Autodesk Inventor part; units mm, degrees
ref_plane "YZ Plane" through (0, 0, 0) normal (1, 0, 0) x (0, 1, 0)
ref_plane "XZ Plane" through (0, 0, 0) normal (0, 1, 0) x (-1, 0, 0)
ref_plane "XY Plane" through (0, 0, 0) normal (0, 0, 1) x (1, 0, 0)
sketch "Szkic1" plane through (0, 0, 0) normal (0, 0, 1) x (1, 0, 0)
  line L0 (0, 0) -> (2.8284, 0)
  line L1 (2.8284, 0) -> (-27.1716, 30)
  line L2 (-27.1716, 30) -> (-27.1716, 27.1716)
  line L3 (-27.1716, 27.1716) -> (0, 0)
  line L4 (-27.1716, 30) -> (-28, 30)
  line L5 (-28, 30) -> (-28, 28)
  line L6 (-28, 28) -> (-27.1716, 28)
  line L7 (-27.1716, 28) -> (-27.1716, 30)
  line L8 (-28, 28) -> (-27.1716, 27.1716)
  dimension "d1" = 30
  dimension "d3" = 45
  dimension "d20" = 2
  dimension "d21" = 2
extrude "Wyciągnięcie proste1" add sketch "Szkic1" along normal blind 196.178
sketch "Szkic4" plane through (-28, 28, 0) normal (-1, 0, 0) x (0, 0, 1)
  line L0 (0, 0) -> (0, -28)
  line L1 (0, 2) -> (196.178, 2)
  line L2 (0, -28) -> (0, 2)
  line L3 (0, 2) -> (30, 2)
  line L4 (30, 2) -> (0, -28)
  line L5 (98.089, 2) -> (98.089, -28) construction
  line L6 (196.178, 0) -> (196.178, -28)
  line L7 (196.178, -28) -> (196.178, 2)
  line L8 (196.178, 2) -> (166.178, 2)
  line L9 (166.178, 2) -> (196.178, -28)
  dimension "d22" = 45
extrude "Wyciągnięcie proste3" cut sketch "Szkic4" against normal through all
sketch "Szkic5" plane through (2.8284, 0, 0) normal (0.7071, 0.7071, 0) x (-0.7071, 0.7071, 0)
  line L0 (41.598, 28) -> (41.598, 168.178) construction
  line L1 (41.598, 98.089) -> (0, 98.089) construction
  line L2 (0, 0) -> (0, 196.178) construction
  point P0 (2, 0)
  point P1 (36.298, 155.089)
  point P2 (36.298, 41.089)
  point P3 (25.298, 167.089)
  point P4 (25.298, 29.089)
  dimension "d25" = 57
  dimension "d26" = 5.3
  dimension "d34" = 69
  dimension "d35" = 16.3
hole "Otwór2" at (-22.8381, 25.6665, 155.089) at (-22.8381, 25.6665, 41.089) at (-15.0599, 17.8884, 167.089) at (-15.0599, 17.8884, 29.089) direction (-0.7071, -0.7071, 0) diameter 3.2 end through all countersink diameter 6.9 countersink angle 84.225
properties part number "Tyl2"
Model file for the job. Use its own axes, mm. Round coordinates to 2 decimals unless told otherwise and drop trailing zeros. Write each loop counter-clockwise with the first axis right and the second up, starting at its lowest first coordinate (ties: lowest second). Pieces come first, ordered by that corner, then holes. Notation, with made-up numbers: (47.25, 8.25) -> (67.25, 8.25) arc R26 cw to (67.25, 44.25) -> close; hole circle Ø3 at (55.5, -30.5). An arc over 180 degrees is marked (long way). Answer as CSV lines item,"result".
1. Slice it at C-C, the plane x = -8.5. List the corners of the cut face in (y, z).
Resolved:
outline,"(8.5, 8.5) -> (11.33, 11.33) -> (11.33, 184.85) -> (8.5, 187.68) -> close"
2. Slice it at A-A, the plane z = 96. List the corners of the cut face in (x, y).
Resolved:
outline,"(-28, 28) -> (0, 0) -> (2.83, 0) -> (-27.17, 30) -> (-28, 30) -> close"
3. Drill centre lines: line 1 (X direction, y = 7.5, z = 112.5); line 2 (X direction, y = 27, z = 63.5); line 3 (Y direction, x = -8.5, z = 31). Where is each one in solid material? Low to high.
Resolved:
line 1,"-7.5 to -4.67"
line 2,"-27 to -24.17"
line 3,"8.5 to 11.33"
4. Slice it at B-B, the plane y = 12.5. List the corners of the cut face in (x, z), plus the area to 3 significant figures.
Resolved:
outline,"(-12.5, 12.5) -> (-9.67, 12.5) -> (-9.67, 183.68) -> (-12.5, 183.68) -> close"
area,"484 mm²"
5. Pin check, flat tips, straight feed: pin 1 Ø12 at (x, z) = (-6.5, 79) entering from -Y; pin 2 Ø4 at (x, z) = (-4, 46.5) entering from -Y; pin 3 Ø3 at (y, z) = (4.5, 117) entering from -X. Stop position of each tip, or through.
Resolved:
pin 1,"y = 0.5"
pin 2,"y = 2"
pin 3,"x = -6"
